Build history of the part. All positions in model axes, mm. A direction names the side the tool comes from. Give positions to 0.01 mm unless a question says otherwise; leave off trailing zeros. Write each loop counter-clockwise with the first axis right and the second up, starting at its lowest first coordinate (ties: lowest second). Pieces come first, ordered by that corner, then holes.
from build123d import *

# Parameters (mm, degrees)
F1_DEPTH = 16
F2_D     = 8


with BuildPart() as f1:
    # F0 (on Front) → F1 (new body)
    with BuildSketch(Plane.XZ):
        with BuildLine():
            Line((-34.6662172288, -19.7492731154), (-35.0371696448, -29.0820410001))
            Line((-35.0371696448, -29.0820410001), (-35.0687167778, -29.8757332816))
            ThreePointArc((-35.0687167778, -29.8757332816), (-26.1158964536, -39.8207528757), (-15.2880338325, -31.9585777605))
            ThreePointArc((-15.2880338325, -31.9585777605), (-13.5435538319, -29.1136706781), (-10.3976923598, -28))
            Line((-10.3976923598, -28), (27.5, -28))
            Line((27.5, -28), (66.2602588043, -28))
            ThreePointArc((66.2602588043, -28), (69.4061202763, -29.1136706781), (71.1506002769, -31.9585777605))
            ThreePointArc((71.1506002769, -31.9585777605), (82.0453345687, -39.8134840129), (90.9303783011, -29.7412059492))
            Line((90.9303783011, -29.7412059492), (90.9089219451, -29.2073580015))
            Line((90.9089219451, -29.2073580015), (90.5287836732, -19.7492731154))
            ThreePointArc((90.5287836732, -19.7492731154), (90.3735319415, -10.1758034804), (93.147096282, -1.0115923959))
            Line((93.147096282, -1.0115923959), (95.278469332, 5.6560345374))
            ThreePointArc((95.278469332, 5.6560345374), (95.5161813728, 11.819450524), (90.1933378417, 14.9357849705))
            Line((90.1933378417, 14.9357849705), (81.4161891549, 14.8464442463))
            ThreePointArc((81.4161891549, 14.8464442463), (79.1559436107, 15.3607918631), (77.3705557582, 16.8391874825))
            ThreePointArc((77.3705557582, 16.8391874825), (75.5074057352, 19.0642678855), (73.4239499151, 21.084545751))
            ThreePointArc((73.4239499151, 21.084545751), (72.7864222514, 21.7553586843), (72.2834406198, 22.5321733286))
            Line((72.2834406198, 22.5321733286), (68.6120607815, 29.5510562145))
            ThreePointArc((68.6120607815, 29.5510562145), (68.0801346369, 31.2567064537), (68.1818484569, 33.0404784292))
            ThreePointArc((68.1818484569, 33.0404784292), (66.351866653, 41.5264608231), (58.5748353368, 45.3837285735))
            Line((58.5748353368, 45.3837285735), (-4.7806569197, 46.1086403504))
            ThreePointArc((-4.7806569197, 46.1086403504), (-12.7004054077, 42.360432851), (-14.6278820787, 33.813134491))
            ThreePointArc((-14.6278820787, 33.813134491), (-14.6773480259, 31.3245006562), (-15.9205954248, 29.168095975))
            Line((-15.9205954248, 29.168095975), (-22.4176771662, 22.5284468379))
            ThreePointArc((-22.4176771662, 22.5284468379), (-23.2975488941, 21.8131223673), (-24.3159760704, 21.3144547002))
            ThreePointArc((-24.3159760704, 21.3144547002), (-26.857680899, 20.2673049491), (-29.284454025, 18.9759652448))
            ThreePointArc((-29.284454025, 18.9759652448), (-30.5179442619, 18.4492237754), (-31.8470764444, 18.2693283014))
            Line((-31.8470764444, 18.2693283014), (-34.7455926018, 18.2693283014))
            ThreePointArc((-34.7455926018, 18.2693283014), (-43.5642704506, 14.4747123862), (-39.7696545355, 5.6560345374))
            Line((-39.7696545355, 5.6560345374), (-37.2845298375, -1.0115923959))
            ThreePointArc((-37.2845298375, -1.0115923959), (-34.510965497, -10.1758034804), (-34.6662172288, -19.7492731154))
        make_face()
        with BuildLine():
            ThreePointArc((0, -18), (-18, 0), (0, 18))
            Line((0, 18), (55, 18))
            ThreePointArc((55, 18), (73, 0), (55, -18))
            Line((55, -18), (0, -18))
        make_face(mode=Mode.SUBTRACT)
    extrude(amount=F1_DEPTH)

    # F2 (through all)
    with Locations(Plane(origin=(0, 0, 0), x_dir=(1, 0, 0), z_dir=(0, 1, 0))):
        with Locations((58.4604231045, -35.3843831029), (-4.8950691519, -36.1092948798), (-25.0687167778, 29.8757332816), (80.9312832222, 29.8757332816)):
            Hole(F2_D / 2)


solid = f1.part
1. Drop flat-ended pins along their axis: pin 1 (8 mm diameter, centred on x = 17, y = -9.5, fed in from +Z); pin 2 (10.5 mm diameter, centred on x = 58.46, z = 35.38, fed in from +Y); pin 3 (2 mm diameter, centred on x = 36.5, y = -8.5, fed in from -Z); pin 4 (2 mm diameter, centred on y = -7.5, z = -3, fed in from +X). Give the stop position or say it passes through.
2. Drill centre lines: line 1 along X through (y, z) = (-2, -1); line 2 along X through (y, z) = (-6.5, -33); line 3 along X through (y, z) = (-14, -34). Where is each one in solid material? Low to high.
3. Saw through at B-B on x = 16. Give the cut face in (y, z).
4. 3-axis set-ups, long thin cutter, end or side, ignore diameter. For faces 4 (the face through (27, -8, 18)), 5 (the face through (69.369, -7.888, -29.084)), 6 (the face through (-19.124, -7.888, 25.895)): which of +Z, -Z, +X, -X, +Y, -Y reach the whole face in a straight line?
5. Mould opens along X. For faces 1 (the face through (-38.544, -7.888, 2.369)), 2 (the face through (-4.374, -8.112, 32.143)), 3 (the face through (68.083, -7.888, 31.232)) say: pulls with the +X half, pulls with the -X half, needs draft (parallel to the pull), parting line crosses it, or undercut.
6. Saw through at A-A on x = 79. Give the cut face in (y, z), plus the area to 3 significant figures.
7. Saw through at C-C on y = -14. Count the separate pieces of the cut face and the enclosed holes in it, plus the area to 3 significant figures.
Outcome:
1. pin 1: stops at z = 45.91
1. pin 2: stops at y = 0
1. pin 3: stops at z = -28
1. pin 4: stops at x = 92.69
2. line 1: x = -37.29 to -17.97, 72.97 to 93.15
2. line 2: x = -34.57 to -27.57, -22.57 to -15.57, 71.43 to 78.43, 83.43 to 90.43
2. line 3: x = -34.18 to -15.96, 71.82 to 90.04
3. outline: (-16, -28) - (0, -28) - (0, -18) - (-16, -18) - close; (-16, 18) - (0, 18) - (0, 45.87) - (-16, 45.87) - close
4. face 4: +Y, -Y
4. face 5: -Z, +Y, -Y
4. face 6: +Z, -X, +Y, -Y
5. face 1: pulls with the -X half
5. face 2: undercut
5. face 3: pulls with the +X half
6. outline: (-16, -39.69) - (0, -39.69) - (0, -33.38) - (-16, -33.38) - close; (-16, -26.37) - (0, -26.37) - (0, 15.44) - (-16, 15.44) - close
6. area: 770 mm2
7. separate pieces: 1
7. enclosed holes: 5
7. area: 5,520 mm2
